Read the model definition and answer for the solid it produces. Units are mm, in the model's axes. A direction names the side the tool comes from. Round coordinates to 2 decimals unless told otherwise and drop trailing zeros. Loops run counter-clockwise (first coordinate to the right, second up) from the corner with the lowest first, then second, coordinate; pieces in that order, holes last. Notation, with made-up numbers: M -17,84.25 L 1,84.25 A35 ccw 1,123.25 Z; hole C 44.25,35 d11. An arc over 180 degrees is marked long. Write each question's results on one line, items separated by ' | '.
from build123d import *

# Parameters (mm, degrees)
ESQUISSE1_W             = 20.2
ESQUISSE1_H             = 15.75
BOSS_EXTRU_1_DEPTH      = 1.5
BOSS_EXTRU_2_DEPTH      = 3.5
BOSS_EXTRU_2_DEPTH_BACK = 1
ESQUISSE2_W             = 18.5
ESQUISSE2_H             = 12
ESQUISSE3_W             = 11.4
ESQUISSE3_H             = 2.2
ENL_V_MAT_EXTRU_1_DEPTH = 13.5
ESQUISSE4_W             = 6
ESQUISSE4_H             = 10.25
BOSS_EXTRU_4_DEPTH      = 5
CHANFREIN1_SIZE         = 1


with BuildPart() as part:
    # Esquisse1 → Boss.-Extru.1 (new body)
    with BuildSketch(Plane(origin=(0, 0, 0), x_dir=(1, 0, 0), z_dir=(0, 1, 0))):
        with Locations((-10.1, 7.875)):
            Rectangle(ESQUISSE1_W, ESQUISSE1_H)
    extrude(amount=BOSS_EXTRU_1_DEPTH)

    # Esquisse2 → Boss.-Extru.2 (add, two sides: drawn at the far end of the back side and taken through both)
    with BuildSketch(Plane(origin=(0, 1.5, 0), x_dir=(1, 0, 0), z_dir=(0, 1, 0)).offset(-BOSS_EXTRU_2_DEPTH_BACK)):
        with Locations((5.75, 7.875)):
            Rectangle(ESQUISSE2_W, ESQUISSE2_H)
    extrude(amount=BOSS_EXTRU_2_DEPTH + BOSS_EXTRU_2_DEPTH_BACK)

    # Esquisse3 → Enlèv. mat.-Extru.1 (cut)
    with BuildSketch(Plane(origin=(15, 0, 0), x_dir=(0, 0, -1), z_dir=(1, 0, 0))):
        with Locations((7.875, 3.6)):
            Rectangle(ESQUISSE3_W, ESQUISSE3_H)
    extrude(amount=-ENL_V_MAT_EXTRU_1_DEPTH, mode=Mode.SUBTRACT)

    # Esquisse4 → Boss.-Extru.4 (add)
    with BuildSketch(Plane(origin=(0, 1.5, 0), x_dir=(1, 0, 0), z_dir=(0, 1, 0))):
        with Locations((-18.7, 4.625)):
            Rectangle(ESQUISSE4_W, ESQUISSE4_H)
    extrude(amount=BOSS_EXTRU_4_DEPTH)

    # Chanfrein1
    # the kernel refuses this chamfer: 1 mm, written as the material it takes off along each edge
    with BuildSketch(Plane(origin=(-13.128317012, 1.5, 0.5), x_dir=(0, -0.02749587661058627, -0.9996219169112968), z_dir=(-1, 0, 0))) as chanfrein1_piece_1_section:
        Polygon((CHANFREIN1_SIZE * 0.999621916911, -CHANFREIN1_SIZE * 0.0274958766106), (-CHANFREIN1_SIZE * 0.0274958766106, -CHANFREIN1_SIZE * 0.999621916911), (0, 0), align=None)
    chanfrein1_piece_1 = extrude(amount=11.143365976, mode=Mode.PRIVATE)
    chanfrein1_piece_1 = split(chanfrein1_piece_1, bisect_by=Plane(origin=(-16.664158506, 1.893401084, 0), z_dir=(0, 0, 1)), keep=Keep.TOP, mode=Mode.PRIVATE)
    chanfrein1_piece_1 = split(chanfrein1_piece_1, bisect_by=Plane(origin=(-20.2, 1.893401084, 0.29176571), z_dir=(1, 0, 0)), keep=Keep.TOP, mode=Mode.PRIVATE)
    add(chanfrein1_piece_1, mode=Mode.SUBTRACT)
    with BuildSketch(Plane(origin=(-13.128317012, 1.5, 0.5), x_dir=(0, -0.02749587661058627, -0.9996219169112968), z_dir=(-1, 0, 0))) as chanfrein1_piece_2_section:
        Polygon((CHANFREIN1_SIZE * 0.999621916911, -CHANFREIN1_SIZE * 0.0274958766106), (-CHANFREIN1_SIZE * 0.0274958766106, -CHANFREIN1_SIZE * 0.999621916911), (0, 0), align=None)
    chanfrein1_piece_2 = extrude(amount=11.143365976, mode=Mode.PRIVATE)
    chanfrein1_piece_2 = split(chanfrein1_piece_2, bisect_by=Plane(origin=(-22.235841494, 1.645570657, 0), z_dir=(0, 0, -1)), keep=Keep.TOP, mode=Mode.PRIVATE)
    chanfrein1_piece_2 = split(chanfrein1_piece_2, bisect_by=Plane(origin=(-20.2, 1.645570657, -0.181859612), z_dir=(-1, 0, 0)), keep=Keep.TOP, mode=Mode.PRIVATE)
    add(chanfrein1_piece_2, mode=Mode.SUBTRACT)
    with BuildSketch(Plane(origin=(-13.128317012, 1.5, 0.5), x_dir=(0, -0.02749587661058627, -0.9996219169112968), z_dir=(-1, 0, 0))) as chanfrein1_piece_3_section:
        Polygon((CHANFREIN1_SIZE * 0.999621916911, -CHANFREIN1_SIZE * 0.0274958766106), (-CHANFREIN1_SIZE * 0.0274958766106, -CHANFREIN1_SIZE * 0.999621916911), (0, 0), align=None)
    chanfrein1_piece_3 = extrude(amount=11.143365976, mode=Mode.PRIVATE)
    chanfrein1_piece_3 = split(chanfrein1_piece_3, bisect_by=Plane(origin=(-22.235841494, 1.893401084, 0), z_dir=(0, 0, 1)), keep=Keep.TOP, mode=Mode.PRIVATE)
    chanfrein1_piece_3 = split(chanfrein1_piece_3, bisect_by=Plane(origin=(-20.2, 1.893401084, 0.29176571), z_dir=(-1, 0, 0)), keep=Keep.TOP, mode=Mode.PRIVATE)
    add(chanfrein1_piece_3, mode=Mode.SUBTRACT)


solid = part.part
Item 1: The part is cut by section D-D (z = -3.75). Determine the outline of the cut face in (x, y).
Outcome:
outline: M -21.7,1.5 L -20.2,1.5 L -20.2,0 L 0,0 L 0,0.5 L 15,0.5 L 15,2.5 L 1.5,2.5 L 1.5,4.7 L 15,4.7 L 15,5 L -3.5,5 L -3.5,1.5 L -15.7,1.5 L -15.7,6.5 L -21.7,6.5 Z
Item 2: The part is cut by section A-A (y = 4). Determine the outline of the cut face in (x, z) (3 decimals).
Outcome:
outline: M -21.7,-9.75 L -15.7,-9.75 L -15.7,0.5 L -21.7,0.5 Z; M -3.5,-13.875 L 15,-13.875 L 15,-13.575 L 1.5,-13.575 L 1.5,-2.175 L 15,-2.175 L 15,-1.875 L -3.5,-1.875 Z
Item 3: The mould has two halves that part along X. Classify faces 1 (the face through (6, 3, -13.875)), 2 (the face through (1.5, 4, -8)), 3 (the face through (-10, 1.5, -8)): pulls with the +X half, pulls with the -X half, needs draft (parallel to the pull), parting line crosses it, or undercut.
Outcome:
face 1: needs draft | face 2: pulls with the +X half | face 3: undercut
Item 4: Flat-ended cylindrical pins translate along their axes: pin 1 (1 mm diameter, centred on x = 6.5, y = 4, fed in from +Z) (3 decimals); pin 2 (1 mm diameter, centred on x = -15.5, y = 4, fed in from -Z); pin 3 (3.5 mm diameter, centred on x = 9, z = -7, fed in from -Y). Find the tip coordinate at first contact, or state that the pin passes through.
Outcome:
pin 1: stops at z = -1.875 | pin 2: stops at z = -9.75 | pin 3: stops at y = 0.5
Item 5: The part is cut by section B-B (x = -1.5). Determine the outline of the cut face in (y, z) (3 decimals), plus the area to 3 significant figures.
Outcome:
outline: M 0,-15.75 L 1.5,-15.75 L 1.5,-13.875 L 5,-13.875 L 5,-1.875 L 1.5,-1.875 L 1.5,0 L 0,0 Z | area: 65.6 mm2
Item 6: The part is cut by section C-C (x = 4). Determine the outline of the cut face in (y, z) (3 decimals).
Outcome:
outline: M 0.5,-13.875 L 5,-13.875 L 5,-1.875 L 0.5,-1.875 Z; hole M 2.5,-13.575 L 4.7,-13.575 L 4.7,-2.175 L 2.5,-2.175 Z
Item 7: Straight lines are drawn through the part: line 1 (Y direction, x = 9, z = -11.25); line 2 (Y direction, x = -19, z = -10.75); line 3 (Z direction, x = 7, y = 2) (3 decimals). For each, find the intervals that lie inside material, in ascending order.
Outcome:
line 1: y = 0.5 to 2.5, 4.7 to 5 | line 2: y = 0 to 1.5 | line 3: z = -13.875 to -1.875
Item 8: For faces 4 (the face through (-19, 4, -9.75)), 5 (the face through (-21, 1.5, -5)), 6 (the face through (8, 2.5, -8)), 7 (the face through (6, 5, -8)), determine the directions among +Z, -Z, +X, -X, +Y, -Y from which every point of the face is accessible in a straight line to the end or side of a thin tool.
Outcome:
face 4: -Z, -X, +Y | face 5: +Z, -Z, -X, -Y | face 6: +X | face 7: +Z, -Z, +X, +Y
